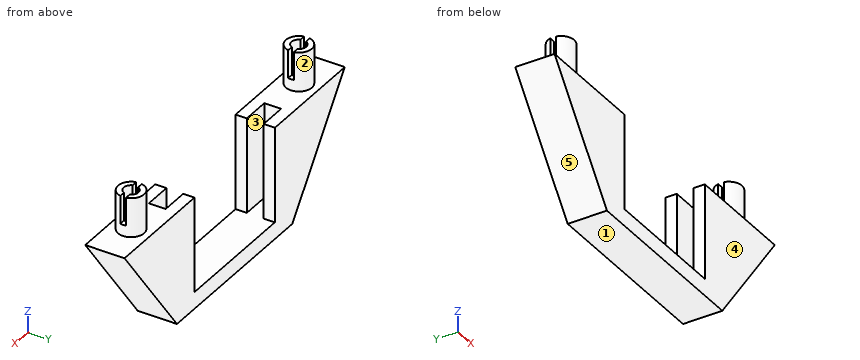
```python
from build123d import *

# Parameters (mm, degrees)
SKETCH1_W           = 33
SKETCH1_H           = 7
BOSS_EXTRUDE1_DEPTH = 3
SKETCH2_W           = 5
SKETCH2_H           = 2
BOSS_EXTRUDE2_DEPTH = 17
BOSS_EXTRUDE3_DEPTH = 7
SKETCH4_R           = 2.325
BOSS_EXTRUDE4_DEPTH = 7
SKETCH5_R           = 1.325
CUT_EXTRUDE1_DEPTH  = 7
SKETCH6_W           = 9.664864402
SKETCH6_H           = 1
SKETCH6_W_2         = 10.163169966
CUT_EXTRUDE2_DEPTH  = 5


with BuildPart() as part:
    # Sketch1 → Boss-Extrude1 (new body)
    with BuildSketch(Plane.XY):
        Rectangle(SKETCH1_W, SKETCH1_H)
    extrude(amount=BOSS_EXTRUDE1_DEPTH)

    # Sketch2 → Boss-Extrude2 (add)
    with BuildSketch(Plane.XY.offset(3)):
        with Locations((-14, 2.5)):
            Rectangle(SKETCH2_W, SKETCH2_H)
        with Locations((-14, -2.5)):
            Rectangle(SKETCH2_W, SKETCH2_H)
        with Locations((14, -2.5)):
            Rectangle(SKETCH2_W, SKETCH2_H)
        with Locations((14, 2.5)):
            Rectangle(SKETCH2_W, SKETCH2_H)
    extrude(amount=BOSS_EXTRUDE2_DEPTH)

    # Sketch3 → Boss-Extrude3 (add)
    with BuildSketch(Plane(origin=(0, 3.5, 0), x_dir=(1, 0, 0), z_dir=(0, 1, 0))):
        Polygon((-16.5, -20), (-31.5, -20), (-16.5, 0), align=None)
        Polygon((16.5, -20), (31.5, -20), (16.5, 0), align=None)
    extrude(amount=-BOSS_EXTRUDE3_DEPTH)

    # Sketch4 → Boss-Extrude4 (add)
    with BuildSketch(Plane.XY.offset(20)):
        with Locations((24, 0)):
            Circle(SKETCH4_R)
        with Locations((-24, 0)):
            Circle(SKETCH4_R)
    extrude(amount=BOSS_EXTRUDE4_DEPTH)

    # Sketch5 → Cut-Extrude1 (cut)
    with BuildSketch(Plane.XY.offset(27)):
        with Locations((-24, 0)):
            Circle(SKETCH5_R)
        with Locations((24, 0)):
            Circle(SKETCH5_R)
    extrude(amount=-CUT_EXTRUDE1_DEPTH, mode=Mode.SUBTRACT)

    # Sketch6 → Cut-Extrude2 (cut)
    with BuildSketch(Plane.XY.offset(27)):
        with Locations((-26.325, 0)):
            Rectangle(SKETCH6_W, SKETCH6_H)
        with Locations((26.325, 0)):
            Rectangle(SKETCH6_W_2, SKETCH6_H)
    extrude(amount=-CUT_EXTRUDE2_DEPTH, mode=Mode.SUBTRACT)


solid = part.part
```
For this review, take the finished solid that the model builds, in its own axes (mm). Face numbers are marked on the shaded views. A direction names the side the tool comes from. Coordinates: 2 decimals unless noted, no trailing zeros. Loops run counter-clockwise (first coordinate to the right, second up) from the corner with the lowest first, then second, coordinate; pieces in that order, holes last.
1. For the marked faces 1 and 2, list the 3-axis set-ups (+Z, -Z, +X, -X, +Y, -Y) from which the entire face can be reached by the end or side of a thin tool; tool diameter is ignored.
2. Add section B-B, the plane z = 24.25. Give the boundary of the cut face in (x, y) (3 decimals), then the cut area to 3 significant figures.
3. Add section C-C, the plane x = 24. Give the boundary of the cut face in (y, z) (3 decimals).
4. Add section A-A, the plane z = 10. Give the boundary of the cut face in (x, y), then the cut area to 3 significant figures.
5. Add section D-D, the plane z = 17.5. Give the boundary of the cut face in (x, y) (3 decimals), then the cut area to 3 significant figures.
6. Mouldability with a two-part tool opening along X and no side actions: class the marked faces 3, 4 and 5 as +X half, -X half, draft (parallel to the pull), parting line (faces both ways), or undercut.
7. Insertion check: P1, Ø0.5, axis at x = -22, z = 25, coming from the -Y side; P2, Ø1.1, axis at x = 26, z = 24.5, coming from the +Y side; P3, Ø0.8, axis at x = -26, y = 0, coming from the +Z side. Each pin has a flat end and moves straight along its axis. Give the tip position at first contact, or say it passes through.
8. For line 1 (X direction, y = 0, z = 21.5) (3 decimals); line 2 (Y direction, x = -24, z = 25.5) (3 decimals); line 3 (Z direction, x = -3.5, y = 2.75), list the stretches that pass through material, from the lowest coordinate up.
Result:
1. face 1: -Z, +X, -X, +Y, -Y
1. face 2: +Z
2. outline: (-26.271, -0.5) arc R2.325 ccw to (-21.729, -0.5) - (-22.773, -0.5) arc R1.325 cw to (-25.227, -0.5) - close; (-26.271, 0.5) - (-25.227, 0.5) arc R1.325 cw to (-22.773, 0.5) - (-21.729, 0.5) arc R2.325 ccw to start; (21.729, -0.5) arc R2.325 ccw to (26.271, -0.5) - (25.227, -0.5) arc R1.325 cw to (22.773, -0.5) - close; (21.729, 0.5) - (22.773, 0.5) arc R1.325 cw to (25.227, 0.5) - (26.271, 0.5) arc R2.325 ccw to start
2. area: 18.9 mm2
3. outline: (-3.5, 10) - (3.5, 10) - (3.5, 20) - (2.325, 20) - (2.325, 27) - (1.325, 27) - (1.325, 20) - (-1.325, 20) - (-1.325, 27) - (-2.325, 27) - (-2.325, 20) - (-3.5, 20) - close
4. outline: (-24, -3.5) - (-11.5, -3.5) - (-11.5, -1.5) - (-16.5, -1.5) - (-16.5, 1.5) - (-11.5, 1.5) - (-11.5, 3.5) - (-24, 3.5) - close; (11.5, -3.5) - (24, -3.5) - (24, 3.5) - (11.5, 3.5) - (11.5, 1.5) - (16.5, 1.5) - (16.5, -1.5) - (11.5, -1.5) - close
4. area: 145 mm2
5. outline: (-29.625, -3.5) - (-11.5, -3.5) - (-11.5, -1.5) - (-16.5, -1.5) - (-16.5, 1.5) - (-11.5, 1.5) - (-11.5, 3.5) - (-29.625, 3.5) - close; (11.5, -3.5) - (29.625, -3.5) - (29.625, 3.5) - (11.5, 3.5) - (11.5, 1.5) - (16.5, 1.5) - (16.5, -1.5) - (11.5, -1.5) - close
5. area: 224 mm2
6. face 3: undercut
6. face 4: draft
6. face 5: -X half
7. P1: stops at y = -1.53
7. P2: stops at y = 1.82
7. P3: stops at z = 22
8. line 1: x = -26.325 to -25.325, -22.675 to -21.675, 21.675 to 22.675, 25.325 to 26.325
8. line 2: y = -2.325 to -1.325, 1.325 to 2.325
8. line 3: z = 0 to 3
